The model under review builds one solid part; all positions refer to its coordinate system, in mm. Face numbers are marked on the shaded views. A direction names the side the tool comes from. Coordinates: 2 decimals unless noted, no trailing zeros. Order: outer loops, then holes, each group sorted by start corner. A loop starts at its lowest first (then second) coordinate and runs counter-clockwise, first axis right, second up. Notation, with made-up numbers: M 51.25,-26 L 76.25,-26 A34 ccw 76.25,6 Z; hole C -8.5,-0.5 d10. An arc over 180 degrees is marked long. Answer in a Markdown table with one row per item.
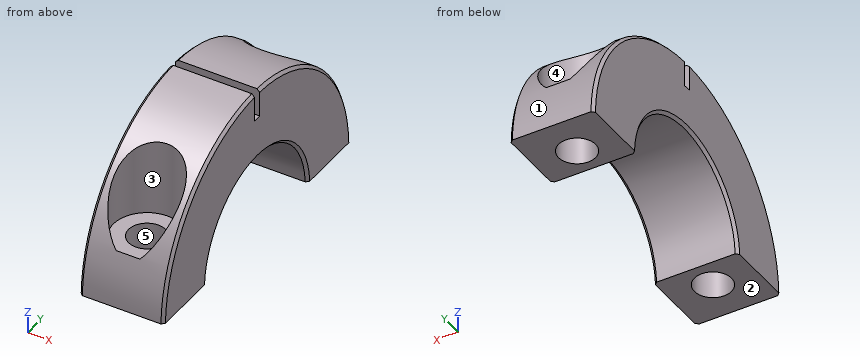
from build123d import *

# Parameters (mm, degrees)
BOSS_EXTRUDE1_DEPTH                     = 15
CUT_EXTRUDE1_DEPTH                      = 42.676582154
CUT_EXTRUDE2_DEPTH                      = 42.669833213
CBORE_FOR_M6_HEX_HEAD_BOLT1_D           = 6.6
CBORE_FOR_M6_HEX_HEAD_BOLT1_CBORE_D     = 12
CBORE_FOR_M6_HEX_HEAD_BOLT1_CBORE_DEPTH = 13.669600757
CHAMFER1_SIZE                           = 0.5


with BuildPart() as part:
    # Sketch1 → Boss-Extrude1 (new body)
    with BuildSketch(Plane(origin=(-7.5, 0, 0), x_dir=(0, -1, 0), z_dir=(-1, 0, 0))):
        with BuildLine():
            Line((-27.489770825, 0.75), (27.489770825, 0.75))
            ThreePointArc((27.489770825, 0.75), (0, 27.5), (-27.489770825, 0.75))
        make_face()
    extrude(amount=-BOSS_EXTRUDE1_DEPTH)

    # Sketch2 → Cut-Extrude1 (cut, through all)
    with BuildSketch(Plane(origin=(7.5, 0, 0), x_dir=(0, 0, -1), z_dir=(1, 0, 0))):
        with BuildLine():
            Line((-27.489770825, -0.75), (-22.5, -0.75))
            Line((-22.5, -0.75), (-22.5, 0.75))
            Line((-22.5, 0.75), (-27.489770825, 0.75))
            ThreePointArc((-27.489770825, 0.75), (-27.5, 0), (-27.489770825, -0.75))
        make_face()
    extrude(amount=-CUT_EXTRUDE1_DEPTH, mode=Mode.SUBTRACT)

    # Sketch3 → Cut-Extrude2 (cut, through all)
    with BuildSketch(Plane(origin=(7.5, 0, 0), x_dir=(0, 0, -1), z_dir=(1, 0, 0))):
        with BuildLine():
            Line((-0.75, -14.981238267), (-0.75, 14.981238267))
            ThreePointArc((-0.75, 14.981238267), (-15, 0), (-0.75, -14.981238267))
        make_face()
    extrude(amount=-CUT_EXTRUDE2_DEPTH, mode=Mode.SUBTRACT)

    # CBORE for M6 Hex Head Bolt1 (through all)
    with Locations(Plane.XY.offset(23.669600757)):
        with Locations((0, -20), (0, 20)):
            CounterBoreHole(CBORE_FOR_M6_HEX_HEAD_BOLT1_D / 2, CBORE_FOR_M6_HEX_HEAD_BOLT1_CBORE_D / 2, CBORE_FOR_M6_HEX_HEAD_BOLT1_CBORE_DEPTH)

    # Chamfer1
    chamfer1_edges = [part.edges().sort_by_distance(p)[0] for p in [
        (7.5, 19.445436483, 19.445436483),
        (-7.5, 0, 15),
        (7.5, 0, 15),
        (-7.5, -19.445436483, 19.445436483),
        (7.5, -19.445436483, 19.445436483),
        (-7.5, 19.445436483, 19.445436483),
    ]]
    chamfer(chamfer1_edges, length=CHAMFER1_SIZE)


solid = part.part
(1) Insertion check: P1, Ø1, axis at x = 4, y = 1.5, coming from the -Z side; P2, Ø4, axis at x = -3, z = 26, coming from the +Y side; P3, Ø1, axis at x = 4.5, y = -17, coming from the +Z side. Each pin has a flat end and moves straight along its axis. Give the tip position at first contact, or say it passes through.
Report:
| item | result |
|---|---|
| P1 | z = 14.87 |
| P2 | y = 13.43 |
| P3 | z = 10 |
(2) Take a section at C-C (y = 0). Write out the cut boundary in (x, z), then the cut area to 3 significant figures.
Report:
| item | result |
|---|---|
| outline | M -7.5,15.5 L -7,15 L 7,15 L 7.5,15.5 L 7.5,22.5 L -7.5,22.5 Z |
| area | 112 mm^2 |
(3) The part is to be moulded in two halves that separate along Y. For the marked faces 1, 2 and 3, say which applies: +Y half, -Y half, draft (parallel to the pull), parting line (faces both ways), or undercut.
Report:
| item | result |
|---|---|
| face 1 | +Y half |
| face 2 | draft |
| face 3 | undercut |
(4) Take a section at B-B (z = 8). State how many separate pieces and enclosed holes the cut face has, then the cut area to 3 significant figures.
Report:
| item | result |
|---|---|
| separate pieces | 2 |
| enclosed holes | 2 |
| area | 339 mm^2 |
(5) Take a section at D-D (x = 5). Write out the cut boundary in (y, z), then the cut area to 3 significant figures.
Report:
| item | result |
|---|---|
| outline | M -27.49,0.75 L -14.98,0.75 A15 cw 14.98,0.75 L 27.49,0.75 A27.5 ccw 23.32,14.58 L 23.32,10 L 16.68,10 L 16.68,21.86 A27.5 ccw 0.75,27.49 L 0.75,22.5 L -0.75,22.5 L -0.75,27.49 A27.5 ccw -16.68,21.86 L -16.68,10 L -23.32,10 L -23.32,14.58 A27.5 ccw Z |
| area | 693 mm^2 |
(6) Machinability: for the marked faces 4 and 5, which of the approach directions +Z, -Z, +X, -X, +Y, -Y give a long, thin tool a straight path to every point of the face, cutting with its end or side? Answer none if there is none.
Report:
| item | result |
|---|---|
| face 4 | +Z |
| face 5 | +Z, -Z |
(7) Take a section at A-A (x = 0). Write out the cut boundary in (y, z).
Report:
| item | result |
|---|---|
| outline | M -27.49,0.75 L -23.3,0.75 L -23.3,10 L -25.62,10 A27.5 ccw Z; M -16.7,0.75 L -14.98,0.75 A15 cw 14.98,0.75 L 16.7,0.75 L 16.7,10 L 14,10 L 14,23.67 A27.5 ccw 0.75,27.49 L 0.75,22.5 L -0.75,22.5 L -0.75,27.49 A27.5 ccw -14,23.67 L -14,10 L -16.7,10 Z; M 23.3,0.75 L 27.49,0.75 A27.5 ccw 25.62,10 L 23.3,10 Z |
(8) To check wall thickness, follow line 1 (Y direction, x = 0, z = 3.25); line 2 (Y direction, x = -2.5, z = 8); line 3 (X direction, y = 20, z = 15). State the ranges of each line that lie inside material, in increasing order. Write a range as [from, to].
Report:
| item | result |
|---|---|
| line 1 | [-27.31, -23.3], [-16.7, -14.64], [14.64, 16.7], [23.3, 27.31] |
| line 2 | [-26.31, -22.15], [-17.85, -12.69], [12.69, 17.85], [22.15, 26.31] |
| line 3 | [-7.5, -6], [6, 7.5] |
